Autodesk Inventor part; units mm, degrees
ref_plane "YZ Plane" through (0, 0, 0) normal (1, 0, 0) x (0, 1, 0)
ref_plane "XZ Plane" through (0, 0, 0) normal (0, 1, 0) x (-1, 0, 0)
ref_plane "XY Plane" through (0, 0, 0) normal (0, 0, 1) x (1, 0, 0)
sketch "Sketch1" plane through (0, 0, 0) normal (0, 0, 1) x (1, 0, 0)
  arc A0 (11.176, 9.652) -> (9.652, 11.176) centre (9.652, 9.652) ccw
  line L0 (11.176, -9.652) -> (11.176, 9.652)
  arc A1 (9.652, -11.176) -> (11.176, -9.652) centre (9.652, -9.652) ccw
  line L1 (-9.652, -11.176) -> (9.652, -11.176)
  arc A2 (-11.176, -9.652) -> (-9.652, -11.176) centre (-9.652, -9.652) ccw
  line L2 (-11.176, 9.652) -> (-11.176, -9.652)
  arc A3 (-9.652, 11.176) -> (-11.176, 9.652) centre (-9.652, 9.652) ccw
  line L3 (9.652, 11.176) -> (-9.652, 11.176)
  arc A4 (-12.7, -10.5918) -> (-10.5918, -12.7) centre (-10.5918, -10.5918) ccw
  line L4 (-10.5918, -12.7) -> (10.5918, -12.7)
  arc A5 (10.5918, -12.7) -> (12.7, -10.5918) centre (10.5918, -10.5918) ccw
  line L5 (12.7, -10.5918) -> (12.7, 10.5918)
  arc A6 (12.7, 10.5918) -> (10.5918, 12.7) centre (10.5918, 10.5918) ccw
  line L6 (10.5918, 12.7) -> (-10.5918, 12.7)
  arc A7 (-10.5918, 12.7) -> (-12.7, 10.5918) centre (-10.5918, 10.5918) ccw
  line L7 (-12.7, 10.5918) -> (-12.7, -10.5918)
  point P0 (0, 0)
extrude "Extrusion1" add sketch "Sketch1" against normal blind 304.8
properties part number "9000"
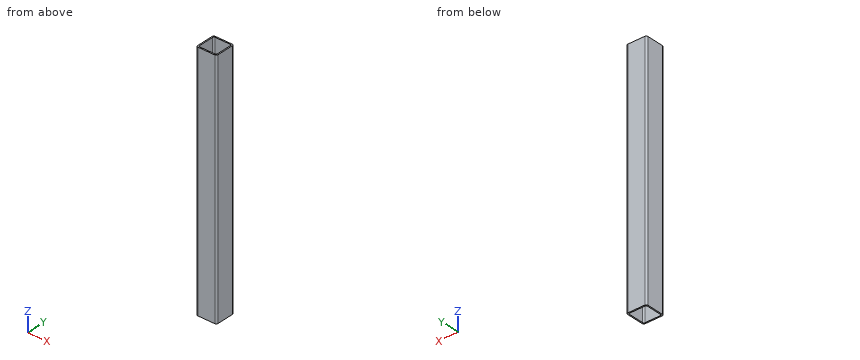
The listing builds one solid part. Answer for the finished solid, in the listing's coordinates (mm). Give positions to 0.01 mm unless a question says otherwise; leave off trailing zeros. Order: outer loops, then holes, each group sorted by start corner. A loop starts at its lowest first (then second) coordinate and runs counter-clockwise, first axis right, second up. Notation, with made-up numbers: (4.25, 8) -> (41.25, 8) arc R21 ccw to (41.25, 21) -> close; hole circle Ø4 at (4.25, -38.75). An arc over 180 degrees is marked (long way). Answer as CSV lines item,"result". Start each with the question number.
Q1. A cutting plane is placed at C-C (z = -179). Determine the outline of the cut face in (x, y).
Q2. A cutting plane is placed at A-A (x = -2). Determine the outline of the cut face in (y, z), then the cut area to 3 significant figures.
Q3. Find the intervals of material crossed by L1, parallel to X at y = -4.25, z = -56.5; L2, parallel to Y at x = 10.75, z = -231, in increasing order.
Results found:
1,outline,"(-12.7, -10.59) arc R2.11 ccw to (-10.59, -12.7) -> (10.59, -12.7) arc R2.11 ccw to (12.7, -10.59) -> (12.7, 10.59) arc R2.11 ccw to (10.59, 12.7) -> (-10.59, 12.7) arc R2.11 ccw to (-12.7, 10.59) -> close; hole (-11.18, -9.65) arc R1.52 ccw to (-9.65, -11.18) -> (9.65, -11.18) arc R1.52 ccw to (11.18, -9.65) -> (11.18, 9.65) arc R1.52 ccw to (9.65, 11.18) -> (-9.65, 11.18) arc R1.52 ccw to (-11.18, 9.65) -> close"
2,outline,"(-12.7, -304.8) -> (-11.18, -304.8) -> (-11.18, 0) -> (-12.7, 0) -> close; (11.18, -304.8) -> (12.7, -304.8) -> (12.7, 0) -> (11.18, 0) -> close"
2,area,"929 mm2"
3,L1,"-12.7 to -11.18, 11.18 to 12.7"
3,L2,"-12.69 to -10.71, 10.71 to 12.69"
